The model under review builds one solid part; all positions refer to its coordinate system, in mm. Coordinates: 2 decimals unless noted, no trailing zeros. Write each loop counter-clockwise with the first axis right and the second up, starting at its lowest first coordinate (ties: lowest second). Pieces come first, ordered by that corner, then holes.
```python
from build123d import *

# Parameters (mm, degrees)
BOSS_EXTRUDE1_DEPTH = 3


with BuildPart() as part:
    # Sketch1 → Boss-Extrude1 (new body)
    with BuildSketch(Plane.XY):
        with BuildLine():
            Line((76.25, -25), (70, -25))
            Line((70, -25), (70, 60))
            Line((70, 60), (74.513154252, 60))
            ThreePointArc((74.513154252, 60), (68.78122292, 68.78122292), (60, 74.513154252))
            ThreePointArc((60, 74.513154252), (58.514821012, 75.039041863), (57, 75.472206616))
            ThreePointArc((57, 75.472206616), (53.899105529, 76.05480457), (50.75, 76.25))
            Line((50.75, 76.25), (-50.75, 76.25))
            ThreePointArc((-50.75, 76.25), (-65.14400917, 71.79904986), (-74.513154252, 60))
            Line((-74.513154252, 60), (-70, 60))
            Line((-70, 60), (-70, -25))
            Line((-70, -25), (-76.25, -25))
            Line((-76.25, -25), (-76.25, -50.75))
            ThreePointArc((-76.25, -50.75), (-68.78122292, -68.78122292), (-50.75, -76.25))
            Line((-50.75, -76.25), (50.75, -76.25))
            ThreePointArc((50.75, -76.25), (68.78122292, -68.78122292), (76.25, -50.75))
            Line((76.25, -50.75), (76.25, -25))
        make_face()
        with BuildLine():
            Line((56.25, -50), (56.25, -47))
            Line((56.25, -47), (49.746794345, -47))
            Line((49.746794345, -47), (36.25, -47))
            Line((36.25, -47), (36.25, -32))
            Line((36.25, -32), (55.669788796, -32))
            Line((55.669788796, -32), (55.669788796, -25))
            Line((55.669788796, -25), (56.25, -25))
            Line((56.25, -25), (62.25, -25))
            Line((62.25, -25), (62.25, 25))
            Line((62.25, 25), (56.249999998, 25))
            Line((56.249999998, 25), (56.249999998, 50.75))
            ThreePointArc((56.249999998, 50.75), (56.102982269, 52.013163019), (55.669788794, 53.208796089))
            Line((55.669788794, 53.208796089), (55.669788794, 56.25))
            Line((55.669788794, 56.25), (-55.669788796, 56.25))
            Line((-55.669788796, 56.25), (-55.669788796, 53.208796089))
            ThreePointArc((-55.669788796, 53.208796089), (-56.10298227, 52.013163019), (-56.25, 50.75))
            Line((-56.25, 50.75), (-56.25, 25))
            Line((-56.25, 25), (-62.25, 25))
            Line((-62.25, 25), (-62.25, -25))
            Line((-62.25, -25), (-56.25, -25))
            Line((-56.25, -25), (-55.669788796, -25))
            Line((-55.669788796, -25), (-55.669788796, -32))
            Line((-55.669788796, -32), (-36.25, -32))
            Line((-36.25, -32), (-36.25, -47))
            Line((-36.25, -47), (-49.746794345, -47))
            Line((-49.746794345, -47), (-56.25, -47))
            Line((-56.25, -47), (-56.25, -50))
            Line((-56.25, -50), (-49.746794345, -50))
            Line((-49.746794345, -50), (49.746794345, -50))
            Line((49.746794345, -50), (56.25, -50))
        make_face(mode=Mode.SUBTRACT)
    extrude(amount=BOSS_EXTRUDE1_DEPTH)


solid = part.part
```
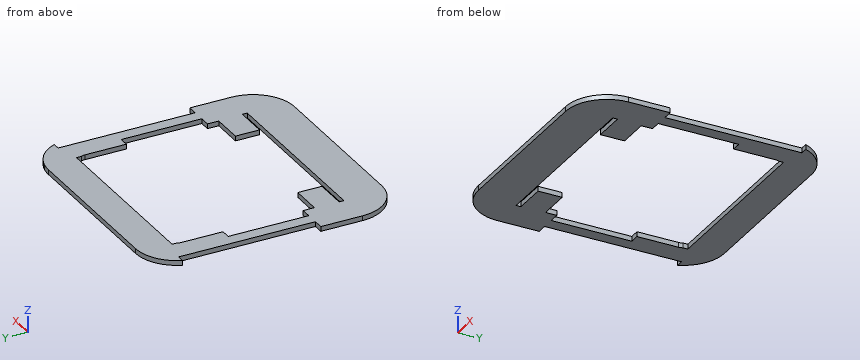
Item 1: To check wall thickness, follow line 1 along Y through (x, z) = (10.5, 0.35); line 2 along X through (y, z) = (20.5, 1); line 3 along X through (y, z) = (40, 0.7). State the ranges of each line that lie inside material, in increasing order.
Solved:
line 1: y = -76.25 to -50, 56.25 to 76.25
line 2: x = -70 to -62.25, 62.25 to 70
line 3: x = -70 to -56.25, 56.25 to 70
Item 2: Take a section at A-A, the plane x = 6.5. Write out the cut boundary in (y, z).
Solved:
outline: (-76.25, 0) - (-50, 0) - (-50, 3) - (-76.25, 3) - close; (56.25, 0) - (76.25, 0) - (76.25, 3) - (56.25, 3) - close
Item 3: For pin 1 (0.9 mm diameter, centred on y = 54, z = 2, fed in from +X); pin 2 (1.5 mm diameter, centred on x = -71.5, z = 1.5, fed in from -Y); pin 3 (0.9 mm diameter, centred on y = 4, z = 2, fed in from -X), all flat-tipped, find the tip position at first contact; note any pin that passes through.
Solved:
pin 1: stops at x = 70
pin 2: stops at y = -66.57
pin 3: stops at x = -70
Item 4: Take a section at C-C, the plane x = 43. Write out the cut boundary in (y, z).
Solved:
outline: (-76.25, 0) - (-50, 0) - (-50, 3) - (-76.25, 3) - close; (-47, 0) - (-32, 0) - (-32, 3) - (-47, 3) - close; (56.25, 0) - (76.25, 0) - (76.25, 3) - (56.25, 3) - close
Item 5: Take a section at B-B, the plane y = -20.5. Write out the cut boundary in (x, z).
Solved:
outline: (-70, 0) - (-62.25, 0) - (-62.25, 3) - (-70, 3) - close; (62.25, 0) - (70, 0) - (70, 3) - (62.25, 3) - close
Item 6: Take a section at D-D, the plane x = 65.5. Write out the cut boundary in (y, z).
Solved:
outline: (-71.55, 0) - (71.55, 0) - (71.55, 3) - (-71.55, 3) - close
